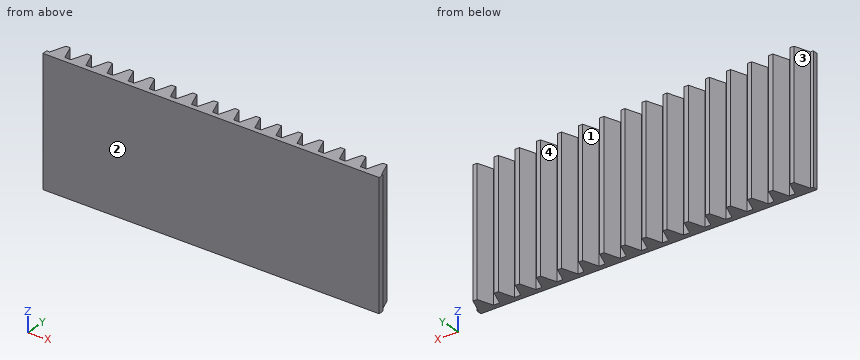
```python
from build123d import *

# Parameters (mm, degrees)
BLANKSKE_W        = 50
BLANKSKE_H        = 3
BLANK_DEPTH       = 19.12
TOOTHCUTSIM_DEPTH = 54.615057586
TEETHCUTS_COUNT   = 17
TEETHCUTS_PITCH   = 3.14159265


with BuildPart() as part:
    # BlankSke → Blank (new body)
    with BuildSketch(Plane.XY):
        with Locations((25, 1.5)):
            Rectangle(BLANKSKE_W, BLANKSKE_H)
    extrude(amount=-BLANK_DEPTH)

    # TooCutSkeSim → ToothCutSim (cut, through all)
    with BuildSketch(Plane.XY):
        Polygon((0.44443537, 0.75), (-0.44443537, 0.75), (-1.272613241, 3.0254), (1.272613241, 3.0254), align=None)
    toothcutsim = extrude(amount=-TOOTHCUTSIM_DEPTH, mode=Mode.SUBTRACT)

    # TeethCuts: ToothCutSim ×17
    with Locations(*[(i * TEETHCUTS_PITCH, 0, 0) for i in range(1, TEETHCUTS_COUNT)]):
        add(toothcutsim, mode=Mode.SUBTRACT)


solid = part.part
```
For this review, take the finished solid that the model builds, in its own axes (mm). Face numbers are marked on the shaded views. Coordinates: 2 decimals unless noted, no trailing zeros. Loops run counter-clockwise (first coordinate to the right, second up) from the corner with the lowest first, then second, coordinate; pieces in that order, holes last. Notation, with made-up numbers: (77, -2.5) -> (83, -2.5) arc R15 ccw to (83, 1.5) -> close; hole circle Ø7 at (11.25, 50.5). An arc over 180 degrees is marked (long way). Return JSON: item names as keys, results as strings. Group by question number.
(1) For pin 1 Ø1.5 at (x, y) = (40, 1) entering from +Z; pin 2 Ø1.5 at (y, z) = (2, -6.5) entering from -X, all flat-tipped, find the tip position at first contact; note any pin that passes through.
(2) To check wall thickness, follow L1, parallel to Y at x = 25, z = -14.5. State the ranges of the line that lie inside material, in increasing order.
(3) Mouldability with a two-part tool opening along X and no side actions: class the marked faces 1, 2, 3 and 4 as pulls with the +X half, pulls with the -X half, needs draft (parallel to the pull), parting line crosses it, or undercut.
(4) Consider section B-B, the plane y = 2.4. Count the separate pieces of the cut face and the enclosed holes in it, plus the area to 3 significant figures.
(5) Consider section A-A, the plane x = 22. Give the boundary of the cut face in (y, z), plus the area to 3 significant figures.
Results below:
{
 "1": {"pin 1": "stops at z = 0", "pin 2": "stops at x = 0.63"},
 "2": {"L1": "y = 0 to 0.75"},
 "3": {"face 1": "undercut", "face 2": "needs draft", "face 3": "pulls with the -X half", "face 4": "undercut"},
 "4": {"separate pieces": "16", "enclosed holes": "0", "area": "322 mm2"},
 "5": {"outline": "(0, -19.12) -> (0.75, -19.12) -> (0.75, 0) -> (0, 0) -> close", "area": "14.3 mm2"}
}
